Read the model definition and answer for the solid it produces. Units are mm, in the model's axes. Face numbers are marked on the shaded views. Round coordinates to 2 decimals unless told otherwise and drop trailing zeros. Order: outer loops, then holes, each group sorted by start corner. A loop starts at its lowest first (then second) coordinate and runs counter-clockwise, first axis right, second up. Notation, with made-up numbers: M -8.5,-12 L 31.5,-12 A13 cw 31.5,12 Z; hole C 51,71.5 d10. An arc over 180 degrees is marked long. Answer as CSV lines item,"result".
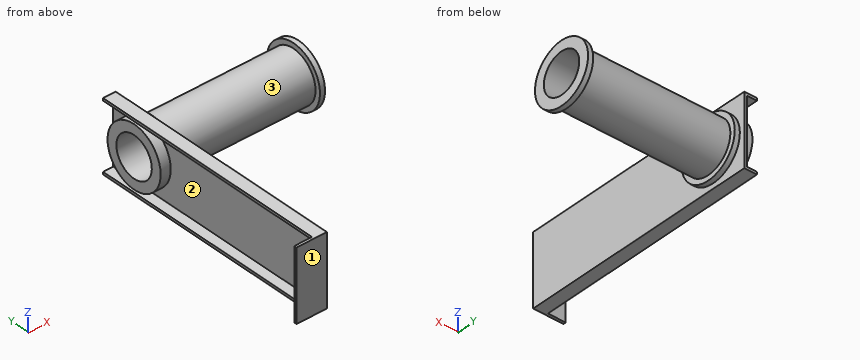
```python
from build123d import *

# Parameters (mm, degrees)
SKETCH1_W           = 44.45
SKETCH1_H           = 149.86
BOSS_EXTRUDE1_DEPTH = 1.5875
SKETCH2_W           = 1.5875
SKETCH2_H           = 149.86
BOSS_EXTRUDE2_DEPTH = 6.35
SKETCH3_W           = 19.05
SKETCH3_H           = 44.45
BOSS_EXTRUDE3_DEPTH = 1.5875
SKETCH4_R           = 19.05
BOSS_EXTRUDE4_DEPTH = 3.175
SKETCH5_R           = 15.875
BOSS_EXTRUDE5_DEPTH = 88.9
SKETCH6_R           = 19.05
BOSS_EXTRUDE6_DEPTH = 3.175
BOSS_EXTRUDE7_START = 6.35
SKETCH7_R           = 19.05
BOSS_EXTRUDE7_DEPTH = 6.35
SKETCH8_R           = 12.7
CUT_EXTRUDE1_DEPTH  = 113.665


with BuildPart() as part:
    # Sketch1 → Boss-Extrude1 (new body)
    with BuildSketch(Plane(origin=(0, 0, 0), x_dir=(0, 0, -1), z_dir=(1, 0, 0))):
        Rectangle(SKETCH1_W, SKETCH1_H)
    extrude(amount=BOSS_EXTRUDE1_DEPTH)

    # Sketch2 → Boss-Extrude2 (add)
    with BuildSketch(Plane.ZY):
        with Locations((21.43125, 0)):
            Rectangle(SKETCH2_W, SKETCH2_H)
        with Locations((-21.43125, 0)):
            Rectangle(SKETCH2_W, SKETCH2_H)
    extrude(amount=BOSS_EXTRUDE2_DEPTH)

    # Sketch3 → Boss-Extrude3 (add)
    with BuildSketch(Plane.XZ.offset(74.93)):
        with Locations((-7.9375, 0)):
            Rectangle(SKETCH3_W, SKETCH3_H)
    extrude(amount=BOSS_EXTRUDE3_DEPTH)

    # Sketch4 → Boss-Extrude4 (add)
    with BuildSketch(Plane(origin=(1.5875, 0, 0), x_dir=(0, 0, -1), z_dir=(1, 0, 0))):
        with Locations(Location((0, 52.705, 0), (0, 0, 180))):
            Circle(SKETCH4_R)
    extrude(amount=BOSS_EXTRUDE4_DEPTH)

    # Sketch5 → Boss-Extrude5 (add)
    with BuildSketch(Plane(origin=(4.7625, 0, 0), x_dir=(0, 0, -1), z_dir=(1, 0, 0))):
        with Locations((0, 52.705)):
            Circle(SKETCH5_R)
    extrude(amount=BOSS_EXTRUDE5_DEPTH)

    # Sketch6 → Boss-Extrude6 (add)
    with BuildSketch(Plane(origin=(93.6625, 0, 0), x_dir=(0, 0, -1), z_dir=(1, 0, 0))):
        with Locations(Location((0, 52.705, 0), (0, 0, 180))):
            Circle(SKETCH6_R)
    extrude(amount=BOSS_EXTRUDE6_DEPTH)

    # Sketch7 → Boss-Extrude7 (add)
    with BuildSketch(Plane.ZY.offset(BOSS_EXTRUDE7_START)):
        with Locations((0, 52.705)):
            Circle(SKETCH7_R)
    extrude(amount=-BOSS_EXTRUDE7_DEPTH)

    # Sketch8 → Cut-Extrude1 (cut)
    with BuildSketch(Plane(origin=(96.8375, 0, 0), x_dir=(0, 0, -1), z_dir=(1, 0, 0))):
        with Locations((0, 52.705)):
            Circle(SKETCH8_R)
    extrude(amount=-CUT_EXTRUDE1_DEPTH, mode=Mode.SUBTRACT)


solid = part.part
```
Item 1: Find the intervals of material crossed by probe 1 along Z at (x, y) = (-6, 11.5) (1 decimal); probe 2 along Y at (x, z) = (36, 0) (3 decimals); probe 3 along X at (y, z) = (36.5, -5), in increasing order. Write a range as [from, to].
Ans:
probe 1,"[-22.2, -20.6], [20.6, 22.2]"
probe 2,"[36.83, 40.005], [65.405, 68.58]"
probe 3,"[-6.35, 4.76], [93.66, 96.84]"
Item 2: A cutting plane is placed at D-D, the plane x = 24.5. Determine the outline of the cut face in (y, z) (3 decimals), and give its area (3 significant figures).
Ans:
outline,"C 52.705,0 d31.75; hole C 52.705,0 d25.4"
area,"285 mm2"
Item 3: Determine the mould class of the marked faces 1, 2 and 3 for opening direction Z: +Z half, -Z half, draft (parallel to the pull), parting line (faces both ways), or undercut.
Ans:
face 1,"draft"
face 2,"undercut"
face 3,"parting line"
Item 4: A cutting plane is placed at C-C, the plane z = 10.5. Determine the outline of the cut face in (x, y).
Ans:
outline,"M -17.46,-76.52 L 1.59,-76.52 L 1.59,36.81 L 4.76,36.81 L 4.76,40.8 L 93.66,40.8 L 93.66,36.81 L 96.84,36.81 L 96.84,45.56 L -6.35,45.56 L -6.35,36.81 L 0,36.81 L 0,-74.93 L -17.46,-74.93 Z; M -6.35,59.85 L 96.84,59.85 L 96.84,68.6 L 93.66,68.6 L 93.66,64.61 L 4.76,64.61 L 4.76,68.6 L 1.59,68.6 L 1.59,74.93 L 0,74.93 L 0,68.6 L -6.35,68.6 Z"
Item 5: Flat-ended cylindrical pins translate along their axes: pin 1 (3 mm diameter, centred on x = 83, z = 2, fed in from +Y); pin 2 (19 mm diameter, centred on y = 58.5, z = 4.5, fed in from +X); pin 3 (4 mm diameter, centred on y = 47.5, z = 8, fed in from +X); pin 4 (8.5 mm diameter, centred on x = -8, z = 9.5, fed in from +Y). Find the tip coordinate at first contact, or state that the pin passes through.
Ans:
pin 1,"y = 68.57"
pin 2,"x = 96.84"
pin 3,"through"
pin 4,"y = 70.92"
